For this review, take the finished solid that the model builds, in its own axes (mm). Face numbers are marked on the shaded views. A direction names the side the tool comes from. Give positions to 0.01 mm unless a question says otherwise; leave off trailing zeros. Write each loop counter-clockwise with the first axis right and the second up, starting at its lowest first coordinate (ties: lowest second). Pieces come first, ordered by that corner, then holes. Notation, with made-up numbers: (-28.5, -10.5) -> (-14.5, -10.5) arc R16 cw to (-14.5, -4.5) -> close; hole circle Ø6 at (31, -23.75). An arc over 180 degrees is marked (long way). Write item = value, one per line.
```python
from build123d import *

# Parameters (mm, degrees)
SKETCH2_R          = 2
CUT_EXTRUDE1_DEPTH = 46.369317826
CIRPATTERN1_COUNT  = 6
SKETCH5_OUTSIDE_W  = 75.336
SKETCH5_OUTSIDE_H  = 75.336
SKETCH5_OUTSIDE_R  = 2
CUT_EXTRUDE2_DEPTH = 10
CIRPATTERN2_COUNT  = 6
SKETCH6_R          = 12
CUT_EXTRUDE3_DEPTH = 4.5
CUT_EXTRUDE4_DEPTH = 15


with BuildPart() as part:
    # Sketch1 → Revolve1 (revolve)
    with BuildSketch(Plane(origin=(0, 0, 0), x_dir=(0, 0, -1), z_dir=(1, 0, 0)), mode=Mode.PRIVATE) as revolve1_sk:
        Polygon((0, 0), (0, 28.25), (5, 28.25), (5, 24.5), (8.5, 24.5), (8.5, 22.5), (26.5, 22.5), (26.5, 0), align=None)
    revolve(revolve1_sk.sketch.rotate(Axis((0, 0, 0), (0, 0, -1)), 90), axis=Axis((0, 0, 0), (0, 0, -1)))

    # Sketch2 → Cut-Extrude1 (cut, symmetric)
    with BuildSketch(Plane(origin=(0, 0, -5), x_dir=(-1, 0, 0), z_dir=(0, 0, -1))):
        with Locations((0, 23.25)):
            Circle(SKETCH2_R)
    cut_extrude1 = extrude(amount=CUT_EXTRUDE1_DEPTH, both=True, mode=Mode.SUBTRACT)

    # CirPattern1: Cut-Extrude1 ×6 about axis
    cirpattern1_axis = Axis((0, 0, 0), (0, 0, 1))
    for i in range(1, CIRPATTERN1_COUNT):
        add(cut_extrude1.rotate(cirpattern1_axis, i * 360 / CIRPATTERN1_COUNT), mode=Mode.SUBTRACT)

    # Sketch5 outside → Cut-Extrude2 (cut)
    # profile 1 of 2: a face of its own
    with BuildSketch(Plane(origin=(0, 0, -26.5), x_dir=(-1, 0, 0), z_dir=(0, 0, -1))):
        Rectangle(SKETCH5_OUTSIDE_W, SKETCH5_OUTSIDE_H)
        with BuildLine():
            ThreePointArc((-1.822401722, 22.426075269), (-11.25, 19.485571585), (-18.510350029, 12.791283822))
            ThreePointArc((-18.510350029, 12.791283822), (-18.40303983, 10.625), (-20.332751751, 9.634791447))
            ThreePointArc((-20.332751751, 9.634791447), (-22.5, 0), (-20.332751751, -9.634791447))
            ThreePointArc((-20.332751751, -9.634791447), (-18.40303983, -10.625), (-18.510350029, -12.791283822))
            ThreePointArc((-18.510350029, -12.791283822), (-11.25, -19.485571585), (-1.822401722, -22.426075269))
            ThreePointArc((-1.822401722, -22.426075269), (0, -21.25), (1.822401722, -22.426075269))
            ThreePointArc((1.822401722, -22.426075269), (11.25, -19.485571585), (18.510350029, -12.791283822))
            ThreePointArc((18.510350029, -12.791283822), (18.40303983, -10.625), (20.332751751, -9.634791447))
            ThreePointArc((20.332751751, -9.634791447), (22.5, 0), (20.332751751, 9.634791447))
            ThreePointArc((20.332751751, 9.634791447), (18.40303983, 10.625), (18.510350029, 12.791283822))
            ThreePointArc((18.510350029, 12.791283822), (11.25, 19.485571585), (1.822401722, 22.426075269))
            ThreePointArc((1.822401722, 22.426075269), (0, 21.25), (-1.822401722, 22.426075269))
        make_face(mode=Mode.SUBTRACT)
    # profile 2 of 2: a face of its own
    with BuildSketch(Plane(origin=(0, 0, -26.5), x_dir=(-1, 0, 0), z_dir=(0, 0, -1))):
        with Locations((0, 17.5)):
            Circle(SKETCH5_OUTSIDE_R)
    cut_extrude2 = extrude(amount=-CUT_EXTRUDE2_DEPTH, mode=Mode.SUBTRACT)

    # CirPattern2: Cut-Extrude2 ×6 about axis
    cirpattern2_axis = Axis((0, 0, 0), (0, 0, 1))
    for i in range(1, CIRPATTERN2_COUNT):
        add(cut_extrude2.rotate(cirpattern2_axis, i * 360 / CIRPATTERN2_COUNT), mode=Mode.SUBTRACT)

    # Sketch6 → Cut-Extrude3 (cut)
    with BuildSketch(Plane.XY):
        Circle(SKETCH6_R)
    extrude(amount=-CUT_EXTRUDE3_DEPTH, mode=Mode.SUBTRACT)

    # Sketch7 → Cut-Extrude4 (cut)
    with BuildSketch(Plane(origin=(0, 0, -26.5), x_dir=(-1, 0, 0), z_dir=(0, 0, -1))):
        with BuildLine():
            ThreePointArc((-1.822401722, 22.426075269), (-11.25, 19.485571585), (-18.510350029, 12.791283822))
            ThreePointArc((-18.510350029, 12.791283822), (-18.40303983, 10.625), (-20.332751751, 9.634791447))
            ThreePointArc((-20.332751751, 9.634791447), (-22.5, 0), (-20.332751751, -9.634791447))
            ThreePointArc((-20.332751751, -9.634791447), (-18.40303983, -10.625), (-18.510350029, -12.791283822))
            ThreePointArc((-18.510350029, -12.791283822), (-11.25, -19.485571585), (-1.822401722, -22.426075269))
            ThreePointArc((-1.822401722, -22.426075269), (0, -21.25), (1.822401722, -22.426075269))
            ThreePointArc((1.822401722, -22.426075269), (11.25, -19.485571585), (18.510350029, -12.791283822))
            ThreePointArc((18.510350029, -12.791283822), (18.40303983, -10.625), (20.332751751, -9.634791447))
            ThreePointArc((20.332751751, -9.634791447), (22.5, 0), (20.332751751, 9.634791447))
            ThreePointArc((20.332751751, 9.634791447), (18.40303983, 10.625), (18.510350029, 12.791283822))
            ThreePointArc((18.510350029, 12.791283822), (11.25, 19.485571585), (1.822401722, 22.426075269))
            ThreePointArc((1.822401722, 22.426075269), (0, 21.25), (-1.822401722, 22.426075269))
        make_face()
    extrude(amount=-CUT_EXTRUDE4_DEPTH, mode=Mode.SUBTRACT)


solid = part.part
```
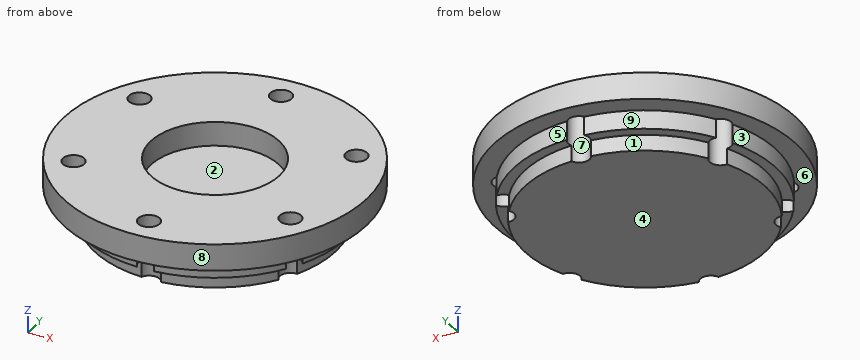
(1) Take a section at C-C (z = -9.75). Write out the cut boundary in (x, y) (3 decimals), plus the area to 3 significant figures.
Answers below:
outline = (-20.333, -9.635) arc R2 cw to (-18.51, -12.791) arc R22.5 ccw to (-1.822, -22.426) arc R2 cw to (1.822, -22.426) arc R22.5 ccw to (18.51, -12.791) arc R2 cw to (20.333, -9.635) arc R22.5 ccw to (20.333, 9.635) arc R2 cw to (18.51, 12.791) arc R22.5 ccw to (1.822, 22.426) arc R2 cw to (-1.822, 22.426) arc R22.5 ccw to (-18.51, 12.791) arc R2 cw to (-20.333, 9.635) arc R22.5 ccw to start
area = 1,570 mm^2
(2) For pin 1 (4 mm diameter, centred on y = -7.5, z = -2.5, fed in from -X); pin 2 (1.3 mm diameter, centred on x = 23, y = -4.5, fed in from -Z); pin 3 (1 mm diameter, centred on x = -18.5, z = -3, fed in from +Y), all flat-tipped, find the tip position at first contact; note any pin that passes through.
Answers below:
pin_1 = -27.71
pin_2 = -8.5
pin_3 = 21.77
(3) Tool access review of the marked faces 1, 2, 3, 4 and 5: name each direction out of +Z, -Z, +X, -X, +Y, -Y from which nothing blocks a thin tool from reaching the whole face with its end or side.
Answers below:
face_1 = -Z, -X, +Y
face_2 = +Z
face_3 = -Z, -X
face_4 = -Z, +X, -X, +Y, -Y
face_5 = -Z, +X, +Y
(4) The part is to be moulded in two halves that separate along X. For the marked faces 6, 7, 8 and 9, say which applies: released by +X, released by -X, zero draft, split by the parting line, or undercut.
Answers below:
face_6 = zero draft
face_7 = undercut
face_8 = split by the parting line
face_9 = released by -X
(5) To check wall thickness, follow probe 1 along Y at (x, z) = (0, -2.7); probe 2 along Z at (x, y) = (-7.5, 4.5); probe 3 along Z at (x, y) = (-6.5, 22). State the ranges of each line that lie inside material, in increasing order.
Answers below:
probe_1 = -28.25 to -25.25, -21.25 to -12, 12 to 21.25, 25.25 to 28.25
probe_2 = -11.5 to -4.5
probe_3 = -8.5 to 0
(6) Take a section at D-D (y = 0). Write out the cut boundary in (x, z).
Answers below:
outline = (-28.25, -5) -> (-24.5, -5) -> (-24.5, -8.5) -> (-22.5, -8.5) -> (-22.5, -11.5) -> (22.5, -11.5) -> (22.5, -8.5) -> (24.5, -8.5) -> (24.5, -5) -> (28.25, -5) -> (28.25, 0) -> (12, 0) -> (12, -4.5) -> (-12, -4.5) -> (-12, 0) -> (-28.25, 0) -> close
(7) Take a section at A-A (x = 0). Write out the cut boundary in (y, z), plus the area to 3 significant figures.
Answers below:
outline = (-28.25, -5) -> (-25.25, -5) -> (-25.25, 0) -> (-28.25, 0) -> close; (-21.25, -11.5) -> (21.25, -11.5) -> (21.25, 0) -> (12, 0) -> (12, -4.5) -> (-12, -4.5) -> (-12, 0) -> (-21.25, 0) -> close; (25.25, -5) -> (28.25, -5) -> (28.25, 0) -> (25.25, 0) -> close
area = 411 mm^2
(8) Take a section at B-B (y = 23.25). Write out the cut boundary in (x, z).
Answers below:
outline = (-16.05, -5) -> (-7.73, -5) -> (-7.73, -8.5) -> (-2, -8.5) -> (-2, 0) -> (-16.05, 0) -> close; (2, -8.5) -> (7.73, -8.5) -> (7.73, -5) -> (16.05, -5) -> (16.05, 0) -> (2, 0) -> close
